Design review of the part built by this model. Coordinates are the model's own, in mm. Give positions to 0.01 mm unless a question says otherwise; leave off trailing zeros. Write each question's results on one line, items separated by ' | '.
from build123d import *

# Parameters (mm, degrees)
SKETCH1_R           = 2.667
BOSS_EXTRUDE1_DEPTH = 6.35


with BuildPart() as part:
    # Sketch1 → Boss-Extrude1 (new body)
    with BuildSketch(Plane(origin=(0, 0, 0), x_dir=(1, 0, 0), z_dir=(0, 1, 0))):
        with BuildLine():
            Line((-273.05, 226.06), (-273.05, 212.09))
            ThreePointArc((-273.05, 212.09), (-272.306051224, 210.293948776), (-270.51, 209.55))
            Line((-270.51, 209.55), (-262.89, 209.55))
            ThreePointArc((-262.89, 209.55), (-261.093948776, 208.806051224), (-260.35, 207.01))
            Line((-260.35, 207.01), (-260.35, 186.69))
            ThreePointArc((-260.35, 186.69), (-261.093948776, 184.893948776), (-262.89, 184.15))
            Line((-262.89, 184.15), (-270.51, 184.15))
            ThreePointArc((-270.51, 184.15), (-272.306051224, 183.406051224), (-273.05, 181.61))
            Line((-273.05, 181.61), (-273.05, -181.61))
            ThreePointArc((-273.05, -181.61), (-272.306051224, -183.406051224), (-270.51, -184.15))
            Line((-270.51, -184.15), (-262.89, -184.15))
            ThreePointArc((-262.89, -184.15), (-261.093948776, -184.893948776), (-260.35, -186.69))
            Line((-260.35, -186.69), (-260.35, -207.01))
            ThreePointArc((-260.35, -207.01), (-261.093948776, -208.806051224), (-262.89, -209.55))
            Line((-262.89, -209.55), (-270.51, -209.55))
            ThreePointArc((-270.51, -209.55), (-272.306051224, -210.293948776), (-273.05, -212.09))
            Line((-273.05, -212.09), (-273.05, -226.06))
            ThreePointArc((-273.05, -226.06), (-272.306051224, -227.856051224), (-270.51, -228.6))
            Line((-270.51, -228.6), (-66.04, -228.6))
            ThreePointArc((-66.04, -228.6), (-64.243948776, -227.856051224), (-63.5, -226.06))
            Line((-63.5, -226.06), (-63.5, -186.69))
            ThreePointArc((-63.5, -186.69), (-62.756051224, -184.893948776), (-60.96, -184.15))
            Line((-60.96, -184.15), (60.96, -184.15))
            ThreePointArc((60.96, -184.15), (62.756051224, -184.893948776), (63.5, -186.69))
            Line((63.5, -186.69), (63.5, -226.06))
            ThreePointArc((63.5, -226.06), (64.243948776, -227.856051224), (66.04, -228.6))
            Line((66.04, -228.6), (270.51, -228.6))
            ThreePointArc((270.51, -228.6), (272.306051224, -227.856051224), (273.05, -226.06))
            Line((273.05, -226.06), (273.05, -212.09))
            ThreePointArc((273.05, -212.09), (272.306051224, -210.293948776), (270.51, -209.55))
            Line((270.51, -209.55), (262.89, -209.55))
            ThreePointArc((262.89, -209.55), (261.093948776, -208.806051224), (260.35, -207.01))
            Line((260.35, -207.01), (260.35, -186.69))
            ThreePointArc((260.35, -186.69), (261.093948776, -184.893948776), (262.89, -184.15))
            Line((262.89, -184.15), (270.51, -184.15))
            ThreePointArc((270.51, -184.15), (272.306051224, -183.406051224), (273.05, -181.61))
            Line((273.05, -181.61), (273.05, 181.61))
            ThreePointArc((273.05, 181.61), (272.306051224, 183.406051224), (270.51, 184.15))
            Line((270.51, 184.15), (262.89, 184.15))
            ThreePointArc((262.89, 184.15), (261.093948776, 184.893948776), (260.35, 186.69))
            Line((260.35, 186.69), (260.35, 207.01))
            ThreePointArc((260.35, 207.01), (261.093948776, 208.806051224), (262.89, 209.55))
            Line((262.89, 209.55), (270.51, 209.55))
            ThreePointArc((270.51, 209.55), (272.306051224, 210.293948776), (273.05, 212.09))
            Line((273.05, 212.09), (273.05, 226.06))
            ThreePointArc((273.05, 226.06), (272.306051224, 227.856051224), (270.51, 228.6))
            Line((270.51, 228.6), (66.04, 228.6))
            ThreePointArc((66.04, 228.6), (64.243948776, 227.856051224), (63.5, 226.06))
            Line((63.5, 226.06), (63.5, 186.69))
            ThreePointArc((63.5, 186.69), (62.756051224, 184.893948776), (60.96, 184.15))
            Line((60.96, 184.15), (-60.96, 184.15))
            ThreePointArc((-60.96, 184.15), (-62.756051224, 184.893948776), (-63.5, 186.69))
            Line((-63.5, 186.69), (-63.5, 226.06))
            ThreePointArc((-63.5, 226.06), (-64.243948776, 227.856051224), (-66.04, 228.6))
            Line((-66.04, 228.6), (-270.51, 228.6))
            ThreePointArc((-270.51, 228.6), (-272.306051224, 227.856051224), (-273.05, 226.06))
        make_face()
        with Locations((-266.7, 222.25)):
            Circle(SKETCH1_R, mode=Mode.SUBTRACT)
        with Locations((266.7, 222.25)):
            Circle(SKETCH1_R, mode=Mode.SUBTRACT)
        with Locations((-241.3, 222.25)):
            Circle(SKETCH1_R, mode=Mode.SUBTRACT)
        with Locations((241.3, 222.25)):
            Circle(SKETCH1_R, mode=Mode.SUBTRACT)
        with Locations((-266.7, -222.25)):
            Circle(SKETCH1_R, mode=Mode.SUBTRACT)
        with Locations((266.7, -222.25)):
            Circle(SKETCH1_R, mode=Mode.SUBTRACT)
        with Locations((-241.3, -222.25)):
            Circle(SKETCH1_R, mode=Mode.SUBTRACT)
        with Locations((241.3, -222.25)):
            Circle(SKETCH1_R, mode=Mode.SUBTRACT)
    extrude(amount=BOSS_EXTRUDE1_DEPTH)


solid = part.part
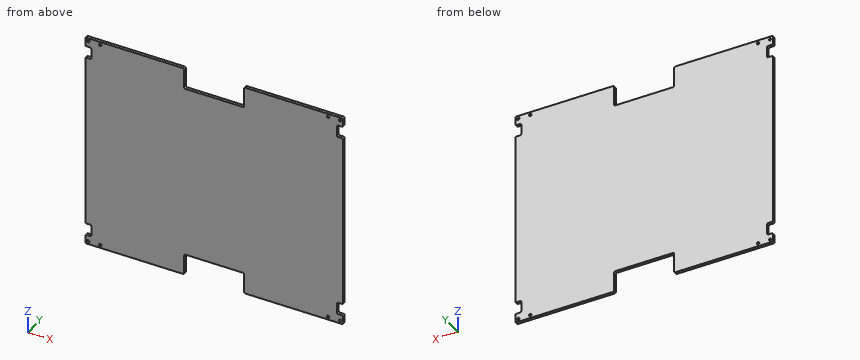
(1) Insertion check: P1, Ø3, axis at y = 3.5, z = -194.5, coming from the +X side; P2, Ø3, axis at y = 4, z = -201.5, coming from the -X side. Each pin has a flat end and moves straight along its axis. Give the tip position at first contact, or say it passes through.
Answers below:
P1: x = 260.35 | P2: x = -260.35
(2) Wall thickness on line 1 along Z through (x, y) = (-241.3, 2.75); line 2 along Z through (x, y) = (-266.7, 4.25); line 3 along X through (y, z) = (4.25, 222.25): over which ranges is each line inside the solid? List them lowest first. Write a range as from..to.
Answers below:
line 1: -228.6..-224.92, -219.58..219.58, 224.92..228.6 | line 2: -228.6..-224.92, -219.58..-209.55, -184.15..184.15, 209.55..219.58, 224.92..228.6 | line 3: -273.05..-269.37, -264.03..-243.97, -238.63..-63.5, 63.5..238.63, 243.97..264.03, 269.37..273.05
(3) Take a section at A-A on y = 3.25. Count the separate pieces of the cut face and the enclosed holes in it, plus the area to 3 significant figures.
Answers below:
separate pieces: 1 | enclosed holes: 8 | area: 237,000 mm2
